Input: part model. Units: mm. Frame: model coordinates. A direction names the side the tool comes from. Coordinates: 2 decimals unless noted, no trailing zeros. Write each loop counter-clockwise with the first axis right and the second up, starting at its lowest first coordinate (ties: lowest second). Pieces come first, ordered by that corner, then holes. Notation, with made-up numbers: M 48.5,62 L 52.5,62 A32 cw 52.5,93 Z; hole C 68,59 d6. An arc over 180 degrees is marked long. Use CSV: the item, a comma, the result in double quotes.
```python
from build123d import *

# Parameters (mm, degrees)
SKETCH1_W           = 237
SKETCH1_H           = 78
BOSS_EXTRUDE1_DEPTH = 48
SKETCH2_W           = 38
SKETCH2_H           = 30
CUT_EXTRUDE1_DEPTH  = 12
CUT_EXTRUDE2_DEPTH  = 150.767319533
SKETCH4_R           = 8
BOSS_EXTRUDE2_DEPTH = 10
BOSS_EXTRUDE3_DEPTH = 6
CUT_EXTRUDE3_DEPTH  = 10
SKETCH7_W           = 2
SKETCH7_H           = 4
BOSS_EXTRUDE4_DEPTH = 10
SKETCH8_W           = 38
SKETCH8_H           = 20
SKETCH8_W_2         = 6
SKETCH8_H_2         = 6
BOSS_EXTRUDE5_DEPTH = 0.5
CUT_EXTRUDE4_DEPTH  = 136.540584451


with BuildPart() as part:
    # Sketch1 → Boss-Extrude1 (new body)
    with BuildSketch(Plane(origin=(0, 0, 0), x_dir=(1, 0, 0), z_dir=(0, 1, 0))):
        Rectangle(SKETCH1_W, SKETCH1_H)
    extrude(amount=BOSS_EXTRUDE1_DEPTH)

    # Sketch2 → Cut-Extrude1 (cut)
    with BuildSketch(Plane(origin=(118.5, 0, 0), x_dir=(0, 0, -1), z_dir=(1, 0, 0))):
        with Locations((-10, 18)):
            Rectangle(SKETCH2_W, SKETCH2_H)
    cut_extrude1 = extrude(amount=-CUT_EXTRUDE1_DEPTH, mode=Mode.SUBTRACT)

    # Sketch3 → Cut-Extrude2 (cut, through all)
    with BuildSketch(Plane.XY.offset(39)):
        with BuildLine():
            Line((118.5, 0), (133.818434768, 0))
            Line((133.818434768, 0), (133.818434768, 98.676655982))
            Line((133.818434768, 98.676655982), (0, 98.676655982))
            Line((0, 98.676655982), (0, 48))
            add(Edge.make_bspline(
                [(118.5, 0), (91.353626717, 83.98617523), (0, 48)],
                knots=[0, 0, 0, 1, 1, 1], degree=2))
        make_face()
    cut_extrude2 = extrude(amount=-CUT_EXTRUDE2_DEPTH, mode=Mode.SUBTRACT)

    # Mirror1: Cut-Extrude1, Cut-Extrude2 across plane
    add(cut_extrude1.mirror(Plane(origin=(0, 0, 0), x_dir=(0, 0, 1), z_dir=(1, 0, 0))), mode=Mode.SUBTRACT)
    add(cut_extrude2.mirror(Plane(origin=(0, 0, 0), x_dir=(0, 0, 1), z_dir=(1, 0, 0))), mode=Mode.SUBTRACT)

    # Sketch4 → Boss-Extrude2 (add)
    with BuildSketch(Plane(origin=(-106.5, 0, 0), x_dir=(0, 0, -1), z_dir=(1, 0, 0))):
        with Locations((-15, 14.792033804)):
            Circle(SKETCH4_R)
    extrude(amount=-BOSS_EXTRUDE2_DEPTH)

    # Sketch5 → Boss-Extrude3 (add)
    with BuildSketch(Plane.XY.offset(39)):
        Polygon((46.5, 35), (38.5, 27), (38.5, 18), (46.5, 10), (80.5, 10), (88.5, 18), (88.5, 27), (80.5, 35), align=None)
    extrude(amount=BOSS_EXTRUDE3_DEPTH)

    # Sketch6 → Cut-Extrude3 (cut)
    with BuildSketch(Plane.XY.offset(45)):
        Polygon((51, 25.5), (56, 30.5), (71, 30.5), (76, 25.5), (76, 14.5), (51, 14.5), align=None)
    extrude(amount=-CUT_EXTRUDE3_DEPTH, mode=Mode.SUBTRACT)

    # Sketch7 → Boss-Extrude4 (add)
    with BuildSketch(Plane.XY.offset(35)):
        with Locations((63.5, 27.549695856)):
            Rectangle(SKETCH7_W, SKETCH7_H)
        with Locations((57.5, 18.950949538)):
            Rectangle(SKETCH7_W, SKETCH7_H)
        with Locations((69.5, 18.950949538)):
            Rectangle(SKETCH7_W, SKETCH7_H)
    extrude(amount=BOSS_EXTRUDE4_DEPTH)

    # Sketch8 → Boss-Extrude5 (add)
    with BuildSketch(Plane.XY.offset(39)):
        with Locations((-61.5, 28)):
            Rectangle(SKETCH8_W, SKETCH8_H)
        with Locations((-86.5, 23.5)):
            Rectangle(SKETCH8_W_2, SKETCH8_H_2)
        with Locations((-86.5, 32.5)):
            Rectangle(SKETCH8_W_2, SKETCH8_H_2)
    extrude(amount=BOSS_EXTRUDE5_DEPTH)

    # Sketch9 → Cut-Extrude4 (cut, through all)
    with BuildSketch(Plane.XZ):
        with BuildLine():
            Line((-112.5, -3), (-118.5, -3))
            Line((-118.5, -3), (-118.5, 3))
            Line((-118.5, 3), (-112.5, 3))
            ThreePointArc((-112.5, 3), (-109.5, 0), (-112.5, -3))
        make_face()
        with BuildLine():
            Line((118.5, 3), (118.5, -3))
            Line((118.5, -3), (112.5, -3))
            ThreePointArc((112.5, -3), (109.5, 0), (112.5, 3))
            Line((112.5, 3), (118.5, 3))
        make_face()
    extrude(amount=-CUT_EXTRUDE4_DEPTH, mode=Mode.SUBTRACT)


solid = part.part
```
1. Section B-B (x = 16.5). Return loops of the section in (y, z), then the cut area to 3 significant figures.
Resolved:
outline,"M 0,-39 L 48,-39 L 48,39 L 0,39 Z"
area,"3,740 mm^2"
2. Material intervals for line 1 (Y direction, x = 52, z = 37); line 2 (Z direction, x = -15, y = 21); line 3 (X direction, y = 3.5, z = 25.5), sorted ascending. Write a range as [from, to].
Resolved:
line 1,"y = [0, 14.5], [26.5, 48]"
line 2,"z = [-39, 39]"
line 3,"x = [-106.5, 106.5]"
3. Section A-A (x = -71). Return loops of the section in (y, z).
Resolved:
outline,"M 0,-39 L 48,-39 L 48,39 L 38,39 L 38,39.5 L 18,39.5 L 18,39 L 0,39 Z"
4. Mould query, pull axis Y, two halves, no side actions, for faces 1 (the flat face through (84.6, 30.9, 42)), 2 (the flat face through (88.5, 22, 42)), 3 (the flat face through (73.5, 28, 40.1)). Classes: pulls with the +Y half, pulls with the -Y half, needs draft (parallel to the pull), parting line crosses it, or undercut.
Resolved:
face 1,"pulls with the +Y half"
face 2,"needs draft"
face 3,"undercut"
5. Access query for faces 4 (the flat face through (64, 14.5, 40)), 5 (the flat face through (-111, 12, 29)), 6 (the flat face through (-106.5, 15, 6)), 7 (the flat face through (63, 31, 45)). Directions: +Z, -Z, +X, -X, +Y, -Y. A direction counts if a zero-diameter tool reaches every point of the face in a straight line with its end or side. Return the directions, or none.
Resolved:
face 4,"+Z"
face 5,"-X, +Y"
face 6,"-X"
face 7,"+Z, +X, -X, +Y, -Y"
6. Contact query for flat-ended pins moving along their axis: pin 1 Ø5 at (y, z) = (22.5, 40.5) entering from -X; pin 2 Ø11 at (y, z) = (22, 41.5) entering from -X; pin 3 Ø9 at (x, y) = (-113, 14) entering from +Z. Output: stop coordinate, or through.
Resolved:
pin 1,"stops at x = -109.99"
pin 2,"stops at x = -111.71"
pin 3,"stops at z = 39"
